```python
from build123d import *

# Parameters (mm, degrees)
ESQUISSE1_W                   = 270
ESQUISSE1_H                   = 213
BOSS_EXTRU_1_DEPTH            = 6
ESQUISSE3_R                   = 9.45
ESQUISSE3_R_2                 = 1.5
ENL_V_MAT_EXTRU_1_DEPTH       = 10
ENL_V_MAT_EXTRU_11_DEPTH      = 173.055950202
ENL_V_MAT_EXTRU_11_DEPTH_BACK = 173.055950202
ESQUISSE6_W                   = 40
ESQUISSE6_H                   = 6
BOSS_EXTRU_2_DEPTH            = 6
ESQUISSE7_W                   = 6
ESQUISSE7_H                   = 30
ESQUISSE7_H_2                 = 27
ENL_V_MAT_EXTRU_12_DEPTH      = 6
ESQUISSE8_W                   = 30
ESQUISSE8_H                   = 6
BOSS_EXTRU_3_DEPTH            = 6
ENL_V_MAT_EXTRU_13_DEPTH      = 176.833017377
ENL_V_MAT_EXTRU_14_DEPTH      = 10
ESQUISSE11_W                  = 6
ESQUISSE11_H                  = 15
ENL_V_MAT_EXTRU_15_DEPTH      = 176.833017377
ENL_V_MAT_EXTRU_17_DEPTH      = 176.833017377
ESQUISSE15_R                  = 2.995
ESQUISSE15_R_2                = 2.95
ESQUISSE15_R_3                = 3
ENL_V_MAT_EXTRU_19_DEPTH      = 3
ESQUISSE16_R                  = 1.5
ENL_V_MAT_EXTRU_20_DEPTH      = 10
ESQUISSE17_W                  = 20
ESQUISSE17_H                  = 6
ENL_V_MAT_EXTRU_22_DEPTH      = 10


with BuildPart() as part:
    # Esquisse1 → Boss.-Extru.1 (new body)
    with BuildSketch(Plane.XY):
        Rectangle(ESQUISSE1_W, ESQUISSE1_H)
    extrude(amount=BOSS_EXTRU_1_DEPTH)

    # Esquisse3 → Enlèv. mat.-Extru.1 (cut)
    with BuildSketch(Plane.XY.offset(6)):
        with Locations((-100, -21.5)):
            Circle(ESQUISSE3_R)
        with Locations((43.489676576, 9.523710062)):
            Circle(ESQUISSE3_R_2)
        with Locations((52.149930614, 4.523710062)):
            Circle(ESQUISSE3_R_2)
        with Locations((35.989676576, -3.466670994)):
            Circle(ESQUISSE3_R_2)
        with Locations((44.649930614, -8.466670994)):
            Circle(ESQUISSE3_R_2)
        with Locations((63.702489497, -19.466670994)):
            Circle(ESQUISSE3_R_2)
        with Locations((72.362743535, -24.466670994)):
            Circle(ESQUISSE3_R_2)
        with Locations((79.862743535, -11.476289938)):
            Circle(ESQUISSE3_R_2)
        with Locations((71.202489497, -6.476289938)):
            Circle(ESQUISSE3_R_2)
    extrude(amount=-ENL_V_MAT_EXTRU_1_DEPTH, mode=Mode.SUBTRACT)

    # Esquisse5 → Enlèv. mat.-Extru.11 (cut, two sides: drawn at the far end of the back side and taken through both)
    with BuildSketch(Plane.XY.offset(6).offset(-ENL_V_MAT_EXTRU_11_DEPTH_BACK)):
        Polygon((135, -36.5), (53.963742643, -43.589753853), (-55, -106.5), (135, -106.5), align=None)
    extrude(amount=ENL_V_MAT_EXTRU_11_DEPTH + ENL_V_MAT_EXTRU_11_DEPTH_BACK, mode=Mode.SUBTRACT)

    # Esquisse6 → Boss.-Extru.2 (add)
    with BuildSketch(Plane(origin=(0, 106.5, 0), x_dir=(1, 0, 0), z_dir=(0, 1, 0))):
        with Locations((-75, -3)):
            Rectangle(ESQUISSE6_W, ESQUISSE6_H)
        with Locations((5, -3)):
            Rectangle(ESQUISSE6_W, ESQUISSE6_H)
        with Locations((85, -3)):
            Rectangle(ESQUISSE6_W, ESQUISSE6_H)
    extrude(amount=BOSS_EXTRU_2_DEPTH)

    # Esquisse7 → Enlèv. mat.-Extru.12 (cut)
    with BuildSketch(Plane(origin=(0, 0, 0), x_dir=(-1, 0, 0), z_dir=(0, 0, -1))):
        with Locations((-132, 91.5)):
            Rectangle(ESQUISSE7_W, ESQUISSE7_H)
        with Locations((-132, 34)):
            Rectangle(ESQUISSE7_W, ESQUISSE7_H_2)
        with Locations((-132, -17)):
            Rectangle(ESQUISSE7_W, ESQUISSE7_H_2)
    extrude(amount=-ENL_V_MAT_EXTRU_12_DEPTH, mode=Mode.SUBTRACT)

    # Esquisse8 → Boss.-Extru.3 (add)
    with BuildSketch(Plane.XZ.offset(106.5)):
        with Locations((-95, 3)):
            Rectangle(ESQUISSE8_W, ESQUISSE8_H)
    extrude(amount=BOSS_EXTRU_3_DEPTH)

    # Esquisse9 → Enlèv. mat.-Extru.13 (cut, through all)
    with BuildSketch(Plane(origin=(0, 0, 0), x_dir=(-1, 0, 0), z_dir=(0, 0, -1))):
        Polygon((-110.25, -38.665344422), (-109.727065544, -32.688176234), (-78.422975963, -35.411286132), (-78.863742643, -41.411286132), align=None)
    extrude(amount=-ENL_V_MAT_EXTRU_13_DEPTH, mode=Mode.SUBTRACT)

    # Esquisse10 → Enlèv. mat.-Extru.14 (cut)
    with BuildSketch(Plane(origin=(0, 0, 0), x_dir=(-1, 0, 0), z_dir=(0, 0, -1))):
        Polygon((-32.03555308, -56.25), (-10.384917986, -68.75), (-7.384917986, -63.553847577), (-29.03555308, -51.053847577), align=None)
        Polygon((11.265717109, -81.25), (32.916352203, -93.75), (35.916352203, -88.553847577), (14.265717109, -76.053847577), align=None)
    extrude(amount=-ENL_V_MAT_EXTRU_14_DEPTH, mode=Mode.SUBTRACT)

    # Esquisse11 → Enlèv. mat.-Extru.15 (cut, through all)
    with BuildSketch(Plane(origin=(0, 0, 0), x_dir=(-1, 0, 0), z_dir=(0, 0, -1))):
        with Locations((72, 52)):
            Rectangle(ESQUISSE11_W, ESQUISSE11_H)
        with Locations((72, 83)):
            Rectangle(ESQUISSE11_W, ESQUISSE11_H)
    extrude(amount=-ENL_V_MAT_EXTRU_15_DEPTH, mode=Mode.SUBTRACT)

    # Esquisse13 → Enlèv. mat.-Extru.17 (cut, through all)
    with BuildSketch(Plane(origin=(0, 0, 0), x_dir=(-1, 0, 0), z_dir=(0, 0, -1))):
        Polygon((-129, 76.5), (-129, 106.5), (-105, 106.5), align=None)
    extrude(amount=-ENL_V_MAT_EXTRU_17_DEPTH, mode=Mode.SUBTRACT)

    # Esquisse15 → Enlèv. mat.-Extru.19 (cut)
    with BuildSketch(Plane(origin=(0, 0, 0), x_dir=(-1, 0, 0), z_dir=(0, 0, -1))):
        with Locations((-85, 109.5)):
            Circle(ESQUISSE15_R)
        with Locations((-5, 109.5)):
            Circle(ESQUISSE15_R)
        with Locations((75, 109.5)):
            Circle(ESQUISSE15_R)
        with Locations((1.940399562, -72.401923789)):
            Circle(ESQUISSE15_R)
        with Locations((-65.76712105, -39.571035308)):
            Circle(ESQUISSE15_R)
        with Locations((45.241669751, -97.401923789)):
            Circle(ESQUISSE15_R_2)
        with Locations((-132, 9.551106058)):
            Circle(ESQUISSE15_R)
        with Locations((-132, 61.579483335)):
            Circle(ESQUISSE15_R)
        with Locations((-119.950479753, -34.805202901)):
            Circle(ESQUISSE15_R)
        with Locations((72, 67.5)):
            Circle(ESQUISSE15_R_3)
        with Locations((85, 53)):
            Circle(ESQUISSE15_R_3)
    extrude(amount=-ENL_V_MAT_EXTRU_19_DEPTH, mode=Mode.SUBTRACT)

    # Esquisse16 → Enlèv. mat.-Extru.20 (cut)
    with BuildSketch(Plane(origin=(0, 0, 0), x_dir=(-1, 0, 0), z_dir=(0, 0, -1))):
        with Locations((-5, 109.5)):
            Circle(ESQUISSE16_R)
        with Locations((74.967795866, 109.5)):
            Circle(ESQUISSE16_R)
        with Locations((-85, 109.5)):
            Circle(ESQUISSE16_R)
        with Locations((-132, 61.579483335)):
            Circle(ESQUISSE16_R)
        with Locations((-132, 9.551106058)):
            Circle(ESQUISSE16_R)
        with Locations((-119.950479753, -34.805202901)):
            Circle(ESQUISSE16_R)
        with Locations((-65.76712105, -39.571035308)):
            Circle(ESQUISSE16_R)
        with Locations((1.940399562, -72.401923789)):
            Circle(ESQUISSE16_R)
        with Locations((45.241669751, -97.401923789)):
            Circle(ESQUISSE16_R)
        with Locations((72, 67.5)):
            Circle(ESQUISSE16_R)
        with Locations((85, 53)):
            Circle(ESQUISSE16_R)
        with Locations((93, 102.5)):
            Circle(ESQUISSE16_R)
    extrude(amount=-ENL_V_MAT_EXTRU_20_DEPTH, mode=Mode.SUBTRACT)

    # Esquisse17 → Enlèv. mat.-Extru.22 (cut)
    with BuildSketch(Plane(origin=(0, 0, 0), x_dir=(-1, 0, 0), z_dir=(0, 0, -1))):
        with Locations((105, 53)):
            Rectangle(ESQUISSE17_W, ESQUISSE17_H)
    extrude(amount=-ENL_V_MAT_EXTRU_22_DEPTH, mode=Mode.SUBTRACT)


solid = part.part
```
Can you work these out from the model? Positions are in its coordinate system, mm. A direction names the side the tool comes from. Round coordinates to 2 decimals unless told otherwise and drop trailing zeros. Loops run counter-clockwise (first coordinate to the right, second up) from the corner with the lowest first, then second, coordinate; pieces in that order, holes last. Notation, with made-up numbers: (63.5, -16) -> (98.5, -16) arc R17 cw to (98.5, -12) -> close; hole circle Ø2 at (-30.75, 70.25). An arc over 180 degrees is marked (long way). Answer in a Markdown table with one row per item.
Item 1: Will these pins go through, and if not, where does the flat tip stop? P1, Ø2.5, axis at x = 79.86, y = -11.48, coming from the +Z side; P2, Ø1.8, axis at x = -73, z = 2.5, coming from the -Y side; P3, Ø5, axis at x = -85, y = 53, coming from the -Z side; P4, Ø1.8, axis at x = -45, z = 3.5, coming from the +Y side.
Answer block:
| item | result |
|---|---|
| P1 | through |
| P2 | y = -106.5 |
| P3 | z = 3 |
| P4 | y = 106.5 |
Item 2: Suppose I cut it at C-C, the plane z = 1. Give the number of separate pieces and of enclosed holes in the cut face, plus the area to 3 significant figures.
Answer block:
| item | result |
|---|---|
| separate pieces | 1 |
| enclosed holes | 23 |
| area | 47,300 mm² |
Item 3: We'd pull the mould along Y, two halves only. Please class faces 1 (the flat face through (-2, 27, 0)), 2 (the flat face through (43.153, -49.831, 2.958)), 3 (the flat face through (-3, -71, 3)): released by +Y, released by -Y, zero draft, split by the parting line, or undercut.
Answer block:
| item | result |
|---|---|
| face 1 | zero draft |
| face 2 | released by -Y |
| face 3 | undercut |
Item 4: If I drill on probe 1 along Y at (x, z) = (-97.5, 1.5); probe 2 along Y at (x, z) = (132, 1.3); probe 3 along Y at (x, z) = (66, 2), over which ranges is the centre line in solid material (lowest first)?
Answer block:
| item | result |
|---|---|
| probe 1 | -112.5 to -30.61, -12.39 to 50, 56 to 106.5 |
| probe 2 | -36.76 to -30.5, -3.5 to 6.56, 12.55 to 20.5, 47.5 to 58.58, 64.57 to 76.5 |
| probe 3 | -36.59 to 112.5 |
Item 5: Suppose I cut it at A-A, the plane y = 82. List the corners of the cut face in (x, z) for me.
Answer block:
| item | result |
|---|---|
| outline | (-135, 0) -> (-75, 0) -> (-75, 6) -> (-135, 6) -> close; (-69, 0) -> (124.6, 0) -> (124.6, 6) -> (-69, 6) -> close |
Item 6: Suppose I cut it at B-B, the plane x = -98. List the corners of the cut face in (y, z) for me.
Answer block:
| item | result |
|---|---|
| outline | (-112.5, 0) -> (-30.74, 0) -> (-30.74, 6) -> (-112.5, 6) -> close; (-12.26, 0) -> (50, 0) -> (50, 6) -> (-12.26, 6) -> close; (56, 0) -> (106.5, 0) -> (106.5, 6) -> (56, 6) -> close |
Item 7: On a 3-axis mill with a long thin cutter (end or side, diameter ignored), from which of +Z, -Z, +X, -X, +Y, -Y can I reach the whole of each face in a straight line? I mean faces 4 (the cylindrical face through (-82.79, 55.03, 1.48)), 5 (the flat face through (25, 109, 3)), 6 (the flat face through (132, 47.5, 3)), 7 (the flat face through (-69, 52, 3)). Say none if no direction works.
Answer block:
| item | result |
|---|---|
| face 4 | -Z |
| face 5 | +Z, -Z, +Y |
| face 6 | +Z, -Z, +X |
| face 7 | +Z, -Z |
